The figure shows three views and two pictorial views of one solid part (mm, origin at its lowest corner). Answer the questions. A direction names the side the tool comes from. Round coordinates to 2 decimals unless told otherwise and drop trailing zeros. Write each loop counter-clockwise with the first axis right and the second up, starting at its lowest first coordinate (ties: lowest second). Pieces come first, ordered by that corner, then holes.
Item 1: Find section C-C on y = 11. Give the vertices of the cut face in (x, z).
Item 2: Find the intervals of material crossed by probe 1 along Z at (x, y) = (11, 4.25); probe 2 along X at (y, z) = (4.5, 12.5); probe 3 along Z at (x, y) = (11, 9.75), in increasing order.
Item 3: For a pull along X with two mould halves and no side action, classify the marked faces 4, 5, 6 and 7 as +X half, -X half, draft (parallel to the pull), parting line (faces both ways), or undercut.
Item 4: A tool of negligible diameter and unlimited length cuts with its end or side. For the marked faces 1, 2 and 3, from which of +Z, -Z, +X, -X, +Y, -Y can it reach the whole face along a straight path? Write none if from no direction.
Item 5: Each of these flat-tipped pins is pushed along its axis until it touches: pin 1 (8 mm diameter, centred on x = 4.5, y = 9.5, fed in from -Z); pin 2 (5.5 mm diameter, centred on x = 11, z = 19, fed in from +Y); pin 3 (6 mm diameter, centred on x = 7.5, z = 20, fed in from -Y); pin 4 (7 mm diameter, centred on x = 11, z = 11, fed in from +Y). Where does it stop, or does it pass through?
Item 6: Find section A-A on z = 11. Give the number of separate pieces and of enclosed holes in the cut face, then the cut area to 3 significant figures.
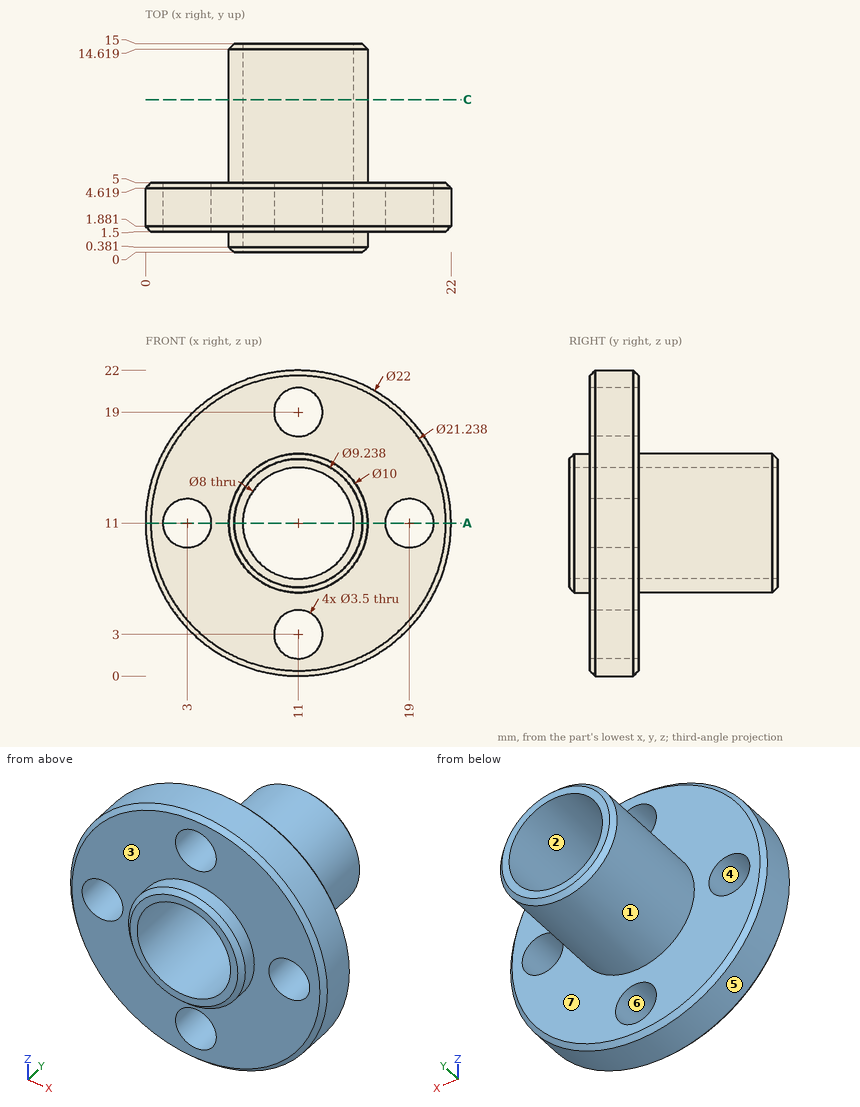
Check values:
1. outline: circle Ø10 at (11, 11); hole circle Ø8 at (11, 11)
2. probe 1: z = 0 to 1.25, 4.75 to 7, 15 to 17.25, 20.75 to 22
2. probe 2: x = 0.1 to 2.1, 3.9 to 7.29, 14.71 to 18.1, 19.9 to 21.9
2. probe 3: z = 6 to 7, 15 to 16
3. face 4: undercut
3. face 5: parting line
3. face 6: undercut
3. face 7: draft
4. face 1: +Y
4. face 2: +Y, -Y
4. face 3: -Y
5. pin 1: stops at z = 6.67
5. pin 2: stops at y = 5
5. pin 3: stops at y = 1.5
5. pin 4: passes through
6. separate pieces: 4
6. enclosed holes: 0
6. area: 46.9 mm2
